from build123d import *

# Parameters (mm, degrees)
SKETCH1_W               = 80.5
SKETCH1_H               = 51.5
BOSS_EXTRUDE1_DEPTH     = 10
SKETCH2_R               = 2.5
CUT_EXTRUDE1_DEPTH      = 11
MIRROR2_COPY_1_SKETCH_R = 2.5
MIRROR2_COPY_1_DEPTH    = 11
SKETCH3_R               = 2.5
CUT_EXTRUDE2_DEPTH      = 11
SKETCH4_R               = 3
CUT_EXTRUDE3_DEPTH      = 11
FILLET1_R               = 2


with BuildPart() as part:
    # Sketch1 → Boss-Extrude1 (new body)
    with BuildSketch(Plane(origin=(0, 0, 0), x_dir=(1, 0, 0), z_dir=(0, 1, 0))):
        Rectangle(SKETCH1_W, SKETCH1_H)
    extrude(amount=BOSS_EXTRUDE1_DEPTH)

    # Sketch2 → Cut-Extrude1 (cut, through all)
    with BuildSketch(Plane(origin=(0, 10, 0), x_dir=(1, 0, 0), z_dir=(0, 1, 0))):
        with Locations((-34.25, 19.25)):
            Circle(SKETCH2_R)
    cut_extrude1 = extrude(amount=-CUT_EXTRUDE1_DEPTH, mode=Mode.SUBTRACT)

    # Mirror1: Cut-Extrude1 across plane
    add(cut_extrude1.mirror(Plane.ZY.offset(20.9)), mode=Mode.SUBTRACT)

    # Mirror2: Cut-Extrude1 across plane
    add(cut_extrude1.mirror(Plane.XY), mode=Mode.SUBTRACT)

    # Mirror2 copy 1 sketch → Mirror2 copy 1 (cut, through all)
    with BuildSketch(Plane(origin=(-41.8, 10, 0), x_dir=(-1, 0, 0), z_dir=(0, 1, 0))):
        with Locations((-34.25, 19.25)):
            Circle(MIRROR2_COPY_1_SKETCH_R)
    extrude(amount=-MIRROR2_COPY_1_DEPTH, mode=Mode.SUBTRACT)

    # Sketch3 → Cut-Extrude2 (cut, through all)
    with BuildSketch(Plane(origin=(0, 10, 0), x_dir=(1, 0, 0), z_dir=(0, 1, 0))):
        with Locations((-20.9, 19.25)):
            Circle(SKETCH3_R)
    extrude(amount=-CUT_EXTRUDE2_DEPTH, mode=Mode.SUBTRACT)

    # Sketch4 → Cut-Extrude3 (cut, through all)
    with BuildSketch(Plane(origin=(0, 10, 0), x_dir=(1, 0, 0), z_dir=(0, 1, 0))):
        with Locations((20.25, -0.45)):
            Circle(SKETCH4_R)
    extrude(amount=-CUT_EXTRUDE3_DEPTH, mode=Mode.SUBTRACT)

    # Fillet1
    fillet1_edges = [part.edges().sort_by_distance(p)[0] for p in [
        (40.25, 5, 25.75),
        (-40.25, 5, 25.75),
        (-40.25, 5, -25.75),
        (40.25, 5, -25.75),
    ]]
    fillet(fillet1_edges, radius=FILLET1_R)


solid = part.part
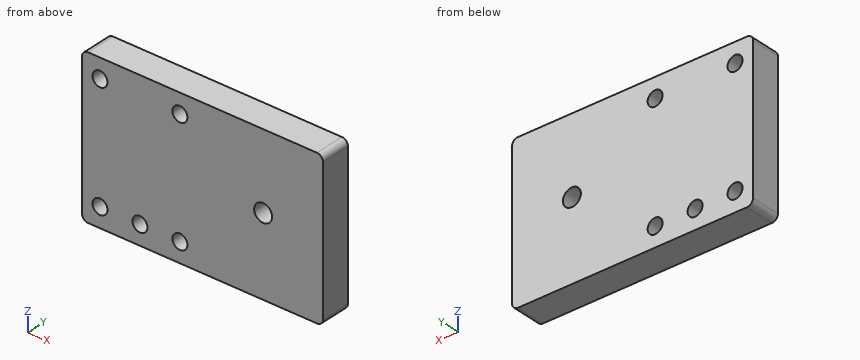
Verification items for the finished model (mm, model axes). Coordinates: 2 decimals unless noted, no trailing zeros. Order: outer loops, then holes, each group sorted by start corner. A loop starts at its lowest first (then second) coordinate and runs counter-clockwise, first axis right, second up. Notation, with made-up numbers: M 42,65.25 L 80,65.25 A8 cw 80,79.25 Z; hole C 14.5,9.5 d9. An arc over 180 degrees is marked long. One line per item, written item: value. Start each with the question number.
Item 1: Thickness scan on probe 1 along X at (y, z) = (7.75, -19.25); probe 2 along Z at (x, y) = (-34.25, 7.5); probe 3 along X at (y, z) = (8.5, -17). Record the ranges inside material, lowest first.
Item 2: Sectioned sample at A-A on z = 19.25. Record the cut outline in (x, y).
Item 3: Sectioned sample at D-D on x = 20.25. Record the cut outline in (y, z).
Item 4: Depth check by flat-ended pin: P1, Ø4, axis at x = -34.25, z = -19.25, coming from the +Y side. Enter the tip coordinate at first touch or a pass-through.
Item 5: Sectioned sample at C-C on z = 0.45. Record the cut outline in (x, y).
Item 6: Sectioned sample at B-B on y = 6.75. Record the cut outline in (x, z).
Calculated:
1. probe 1: -40.25 to -36.75, -31.75 to -23.4, -18.4 to -10.05, -5.05 to 40.25
1. probe 2: -25.75 to -21.75, -16.75 to 16.75, 21.75 to 25.75
1. probe 3: -40.25 to -35.34, -33.16 to -21.99, -19.81 to -8.64, -6.46 to 40.25
2. outline: M -40.25,0 L -36.75,0 L -36.75,10 L -40.25,10 Z; M -31.75,0 L -10.05,0 L -10.05,10 L -31.75,10 Z; M -5.05,0 L 40.25,0 L 40.25,10 L -5.05,10 Z
3. outline: M 0,-25.75 L 10,-25.75 L 10,-2.55 L 0,-2.55 Z; M 0,3.45 L 10,3.45 L 10,25.75 L 0,25.75 Z
4. P1: through
5. outline: M -40.25,0 L 17.25,0 L 17.25,10 L -40.25,10 Z; M 23.25,0 L 40.25,0 L 40.25,10 L 23.25,10 Z
6. outline: M -40.25,-23.75 A2 ccw -38.25,-25.75 L 38.25,-25.75 A2 ccw 40.25,-23.75 L 40.25,23.75 A2 ccw 38.25,25.75 L -38.25,25.75 A2 ccw -40.25,23.75 Z; hole C -34.25,-19.25 d5; hole C -34.25,19.25 d5; hole C -20.9,-19.25 d5; hole C -7.55,-19.25 d5; hole C -7.55,19.25 d5; hole C 20.25,0.45 d6
